Check sheet for the drawn part. Datum: minimum x, y, z corner. Units: mm. Round coordinates to 2 decimals unless told otherwise and drop trailing zeros. Write each loop counter-clockwise with the first axis right and the second up, starting at its lowest first coordinate (ties: lowest second). Pieces come first, ordered by that corner, then holes.
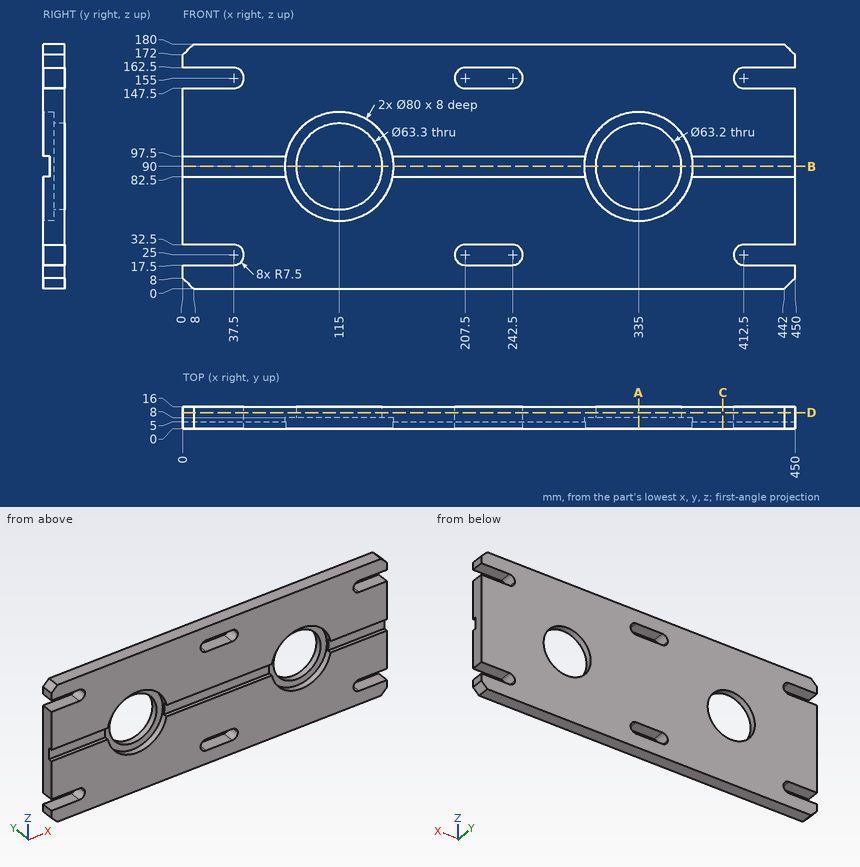
Q1. Material ranges on line 1 along Z through (x, y) = (415.5, 11); line 2 along Z through (x, y) = (115, 11); line 3 along Z through (x, y) = (335, 2), recorded low to high.
Recorded:
line 1: z = 0 to 17.5, 32.5 to 147.5, 162.5 to 180
line 2: z = 0 to 58.35, 121.65 to 180
line 3: z = 0 to 50, 130 to 180
Q2. Sectioned sample at B-B (z = 90). Enter the section's corners in (x, y).
Recorded:
outline: (0, 5) - (75, 5) - (75, 8) - (83.35, 8) - (83.35, 16) - (0, 16) - close; (146.65, 8) - (155, 8) - (155, 5) - (295, 5) - (295, 8) - (303.4, 8) - (303.4, 16) - (146.65, 16) - close; (366.6, 8) - (375, 8) - (375, 5) - (450, 5) - (450, 16) - (366.6, 16) - close
Q3. Sectioned sample at A-A (x = 335). Enter the section's corners in (y, z).
Recorded:
outline: (0, 0) - (16, 0) - (16, 58.4) - (8, 58.4) - (8, 50) - (0, 50) - close; (0, 130) - (8, 130) - (8, 121.6) - (16, 121.6) - (16, 180) - (0, 180) - close
Q4. Depth check by flat-ended pin: P1, Ø7.5, axis at x = 239.5, z = 87.5, coming from the -Y side; P2, Ø1.5, axis at y = 11, z = 151, coming from the +X side. Enter the tip coordinate at first touch or a pass-through.
Recorded:
P1: stops at y = 5
P2: stops at x = 406.7
Q5. Sectioned sample at D-D (y = 11.75). Give the number of separate pieces and of enclosed holes in the cut face, plus the area to 3 significant figures.
Recorded:
separate pieces: 1
enclosed holes: 4
area: 70,600 mm2
Q6. Sectioned sample at C-C (x = 397). Enter the section's corners in (y, z).
Recorded:
outline: (0, 0) - (16, 0) - (16, 180) - (0, 180) - (0, 97.5) - (5, 97.5) - (5, 82.5) - (0, 82.5) - close
